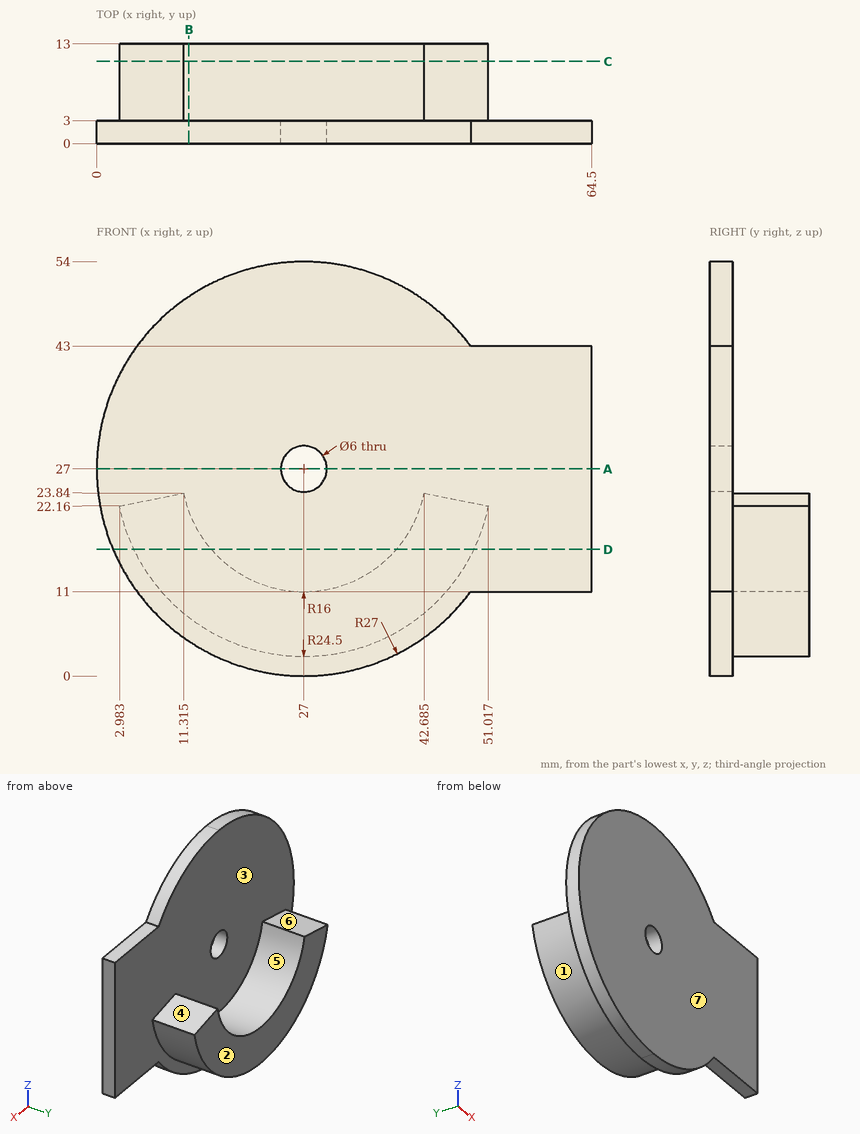
Here's the drawing with two shaded views (mm, measured from the low corner). I have some questions. A direction names the side the tool comes from. Give positions to 0.01 mm unless a question says otherwise; leave off trailing zeros. Loops run counter-clockwise (first coordinate to the right, second up) from the corner with the lowest first, then second, coordinate; pieces in that order, holes last. Notation, with made-up numbers: M 49.5,71.5 L 55.5,71.5 A12 cw 55.5,80.5 Z; hole C -33,-25 d11. An arc over 180 degrees is marked long. Use one line per item in the form item = value. Start each with the question number.
Q1. Will these pins go through, and if not, where does the flat tip stop? pin 1 Ø2.5 at (x, y) = (54, 1.5) entering from -Z; pin 2 Ø5 at (y, z) = (7.5, 21.5) entering from -X; pin 3 Ø16 at (x, z) = (16.5, 31.5) entering from +Y.
Q2. Which directions (+Z, -Z, +X, -X, +Y, -Y) give clear straight access to the entire face, cutting with the end or side of a thin tool? Please do the marked faces 5, 6 and 7.
Q3. If we section it at C-C (y = 10.75): Write out the boundary of the cut face in (x, z) (1 decimal), then the cut area to 3 significant figures.
Q4. If we section it at B-B (x = 12): Write out the boundary of the cut face in (y, z), then the cut area to 3 significant figures.
Q5. If we section it at D-D (z = 16.5): Write out the boundary of the cut face in (x, y) (1 decimal).
Q6. I need wall thicknesses on line 1 along X through (y, z) = (1.7, 27); line 2 along Y through (x, z) = (37.5, 27.5); line 3 along X through (y, z) = (1.5, 28). Which ranges of each line are inside material? Lowest first, please.
Q7. If we section it at A-A (z = 27): Write out the boundary of the cut face in (x, y).
Q8. Thinking about a two-plate mould opening in X: for the marked faces 1, 2, 3 and 4, which applies, +X half, -X half, draft (parallel to the pull), parting line (faces both ways), or undercut?
Taken from the geometry:
q1.pin_1 = 11
q1.pin_2 = 2.98
q1.pin_3 = 3
q2.face_5 = +Z, +Y
q2.face_6 = +Z, -X, +Y
q2.face_7 = +Z, -Z, +X, -X, -Y
q3.outline = M 3,22.2 A24.5 ccw 51,22.2 L 42.7,23.8 A16 cw 11.3,23.8 Z
q3.area = 472 mm^2
q4.outline = M 0,4.55 L 3,4.55 L 3,7.63 L 13,7.63 L 13,21.43 L 3,21.43 L 3,49.45 L 0,49.45 Z
q4.area = 273 mm^2
q5.outline = M 2.1,0 L 64.5,0 L 64.5,3 L 49.1,3 L 49.1,13 L 39.1,13 L 39.1,3 L 14.9,3 L 14.9,13 L 4.9,13 L 4.9,3 L 2.1,3 Z
q6.line_1 = 0 to 24, 30 to 64.5
q6.line_2 = 0 to 3
q6.line_3 = 0.02 to 24.17, 29.83 to 64.5
q7.outline = M 0,0 L 24,0 L 24,3 L 0,3 Z; M 30,0 L 64.5,0 L 64.5,3 L 30,3 Z
q8.face_1 = parting line
q8.face_2 = draft
q8.face_3 = undercut
q8.face_4 = +X half
